Autodesk Inventor part; units mm, degrees
ref_plane "YZ Plane" through (0, 0, 0) normal (1, 0, 0) x (0, 1, 0)
ref_plane "XZ Plane" through (0, 0, 0) normal (0, 1, 0) x (-1, 0, 0)
ref_plane "XY Plane" through (0, 0, 0) normal (0, 0, 1) x (1, 0, 0)
sketch "Sketch1" plane through (0, 0, 0) normal (0, 0, 1) x (1, 0, 0)
  line L0 (0, -8.75) -> (0, 8.75) construction
  line L1 (-8.19, 0) -> (8.19, 0) construction
  line L2 (-5.85, -6.25) -> (5.85, -6.25)
  line L3 (5.85, -6.25) -> (5.85, 6.25)
  line L4 (5.85, 6.25) -> (-5.85, 6.25)
  line L5 (-5.85, 6.25) -> (-5.85, -6.25)
  line L6 (0, -6.25) -> (0, 6.25) construction
  point P0 (0, 0)
  dimension "d0" = 12.5
  dimension "d1" = 11.7
extrude "Extrusion1" add sketch "Sketch1" along normal blind 2.6
sketch "Sketch3" plane through (-5.85, -6.25, 0) normal (-1, 0, 0) x (0, 0, 1)
  line L0 (0, 12.5) -> (0, 0) construction
  line L1 (0, 0) -> (2.6, 0) construction
  circle A0 centre (1.45, 1.15) radius 1.05
  line L2 (1.45, 1.15) -> (2.5, 1.15) construction
  line L3 (2.6, 12.5) -> (2.6, 0) construction
  line L4 (1.45, 1.15) -> (1.45, 0.1) construction
  point P0 (0, 6.25)
  dimension "d10" = 2.1
  dimension "d11" = 0.1
  dimension "d23" = 0.1
extrude "Extrusion3" add sketch "Sketch3" along normal blind 1.4
sketch "Sketch4" plane through (0, 0, 2.6) normal (0, 0, 1) x (1, 0, 0)
  line L0 (-5.85, -6.25) -> (5.85, -6.25) construction
  line L1 (-5.85, 6.25) -> (-5.85, -6.25) construction
  line L2 (-2.25, -6.25) -> (-3.85, -6.25)
  line L3 (-3.85, -6.25) -> (-3.85, 1.75)
  line L4 (-3.85, 1.75) -> (-2.25, 1.75)
  line L5 (-2.25, 1.75) -> (-2.25, -6.25)
  point P0 (0, 0)
  dimension "d18" = 2
  dimension "d19" = 1.6
  dimension "d20" = 8
extrude "Extrusion4" cut sketch "Sketch4" against normal through all
mirror "Mirror1" about plane through (0, 0, 0) normal (1, 0, 0) of "Extrusion3", "Extrusion4"
sketch "Sketch6" plane through (-5.85, -6.25, 0) normal (-1, 0, 0) x (0, 0, 1)
  circle A0 centre (1.45, 1.15) radius 1.05 construction
  line L0 (0, 0) -> (2.6, 0) construction
  line L1 (2.6, 12.5) -> (2.6, 0) construction
  line L2 (0, 12.5) -> (0, 0) construction
  arc A1 (1.45, 0) -> (2.6, 1.15) centre (1.45, 1.15) ccw
  line L3 (1.45, 1.15) -> (2.6, 1.15) construction
  line L4 (1.45, 1.15) -> (1.45, 0) construction
  line L5 (0, 1.25) -> (-2, 1.25)
  line L6 (-2, 1.25) -> (-2, -1.75)
  line L7 (-2, -1.75) -> (3, -1.75)
  line L8 (3, -1.75) -> (3, 1.25)
  line L9 (3, 1.25) -> (2.6, 1.15)
  arc A2 (0, 1.25) -> (1.25, 0) centre (1.25, 1.25) ccw
  line L10 (1.25, 0) -> (1.45, 0)
  line L11 (0.0201, 1.25) -> (1.25, 1.25) construction
  point P0 (0, 6.25)
  point P1 (3, 1.25)
  dimension "d32" = 3
  dimension "d34" = 3
  dimension "d49" = 0.2
  dimension "d50" = 2
  dimension "d51" = 5
extrude "Extrusion5" cut sketch "Sketch6" against normal through all
fillet "Fillet1" radius 0.6 4 edges at (-3.85, 1.75, 1.3) (-2.25, 1.75, 1.3) (3.85, 1.75, 1.3) (2.25, 1.75, 1.3)
fillet "Fillet3" radius 1.2 1 edges at (0, 6.25, 2.6)
properties part number "tilt_leg"
Model file for the job. Use its own axes, mm. A direction names the side the tool comes from. Coordinates: 2 decimals unless noted, no trailing zeros. Write each loop counter-clockwise with the first axis right and the second up, starting at its lowest first coordinate (ties: lowest second). Pieces come first, ordered by that corner, then holes. Notation, with made-up numbers: (58.5, 88) -> (81.5, 88) arc R30 ccw to (81.5, 111) -> close; hole circle Ø6 at (86, -21.75). An arc over 180 degrees is marked (long way). One line per item, written item: value. Start each with the question number.
1) Flat gauge pins, fed straight in: pin 1 Ø1.3 at (y, z) = (-3, 1.5) entering from -X; pin 2 Ø0.8 at (y, z) = (-1.5, 1) entering from +X. Where does each tip first touch, or does it go through?
2) Slice it at D-D on y = 3.5. Write the cut outline in (x, z), then the cut area to 3 significant figures.
3) Pull direction X, two halves, no side cores. Call faces 1 (the face through (5.85, 1, 1)), 2 (the face through (0, 0, 2.6)), 3 (the face through (-3.85, -3, 1)): +X half, -X half, draft (parallel to the pull), parting line (faces both ways), or undercut.
4) Slice it at A-A on y = -2.5. Write the cut outline in (x, z), then the cut area to 3 significant figures.
5) Which spindle directions (+Z, -Z, +X, -X, +Y, -Y) get a long thin tool onto all of the face, cutting with end or side? Do faces 4 (the face through (-0.031, -5.874, 0.356)), 5 (the face through (6.54, -6.125, 1.222)), 6 (the face through (-2.25, -2, 1)), 7 (the face through (-6.54, -4.168, 1.935)). Say none if no direction does.
6) Probe probe 1 along X at (y, z) = (-4.75, 2.15); probe 2 along X at (y, z) = (-3, 1.45); probe 3 along X at (y, z) = (5.25, 1.5). List the from-to ranges inside material, lowest first.
7) Slice it at B-B on x = 0.5. Write the cut outline in (y, z).
8) Slice it at C-C on z = 2.15. Write the cut outline in (x, y).
Answers follow:
1. pin 1: x = -5.85
1. pin 2: x = 5.85
2. outline: (-5.85, 0) -> (5.85, 0) -> (5.85, 2.6) -> (-5.85, 2.6) -> close
2. area: 30.4 mm2
3. face 1: +X half
3. face 2: draft
3. face 3: undercut
4. outline: (-5.85, 0) -> (-3.85, 0) -> (-3.85, 2.6) -> (-5.85, 2.6) -> close; (-2.25, 0) -> (2.25, 0) -> (2.25, 2.6) -> (-2.25, 2.6) -> close; (3.85, 0) -> (5.85, 0) -> (5.85, 2.6) -> (3.85, 2.6) -> close
4. area: 22.1 mm2
5. face 4: -Z, +X, -X, -Y
5. face 5: +X
5. face 6: +Z, -Z, -Y
5. face 7: -X
6. probe 1: -7.25 to -3.85, -2.25 to 2.25, 3.85 to 7.25
6. probe 2: -5.85 to -3.85, -2.25 to 2.25, 3.85 to 5.85
6. probe 3: -5.85 to 5.85
7. outline: (-6.25, 1.25) arc R1.25 ccw to (-5, 0) -> (6.25, 0) -> (6.25, 1.4) arc R1.2 ccw to (5.05, 2.6) -> (-5.1, 2.6) arc R1.15 ccw to (-6.25, 1.45) -> close
8. outline: (-7.25, -5.88) -> (-5.85, -5.88) -> (-5.85, -6.01) -> (-3.85, -6.01) -> (-3.85, 1.15) arc R0.6 cw to (-3.25, 1.75) -> (-2.85, 1.75) arc R0.6 cw to (-2.25, 1.15) -> (-2.25, -6.01) -> (2.25, -6.01) -> (2.25, 1.15) arc R0.6 cw to (2.85, 1.75) -> (3.25, 1.75) arc R0.6 cw to (3.85, 1.15) -> (3.85, -6.01) -> (5.85, -6.01) -> (5.85, -5.88) -> (7.25, -5.88) -> (7.25, -4.32) -> (5.85, -4.32) -> (5.85, 5.99) -> (-5.85, 5.99) -> (-5.85, -4.32) -> (-7.25, -4.32) -> close
